Geometry: final body of the model. Coordinates: model frame, mm. Face numbers are marked on the shaded views. A direction names the side the tool comes from. Round coordinates to 2 decimals unless told otherwise and drop trailing zeros. Write each loop counter-clockwise with the first axis right and the second up, starting at its lowest first coordinate (ties: lowest second). Pieces come first, ordered by that corner, then holes. Notation, with made-up numbers: (41, 7) -> (49, 7) arc R28 ccw to (49, 37) -> close; hole circle Ø8 at (81, 39.25). An arc over 180 degrees is marked (long way). One line per item, written item: value. Start each with the question number.
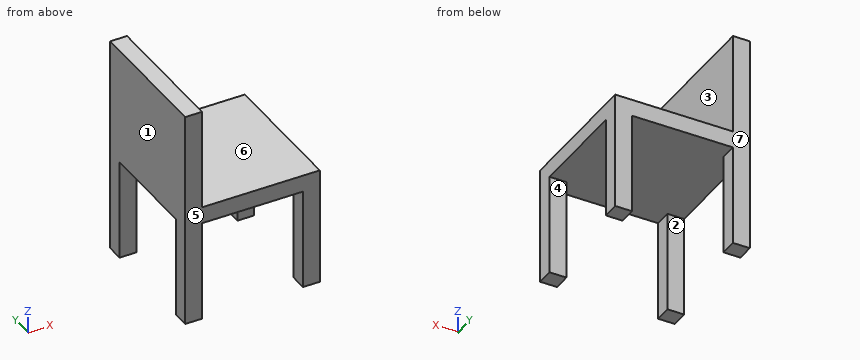
from build123d import *

# Parameters (mm, degrees)
F0_W     = 101.6
F0_H     = 101.6
F1_DEPTH = 12.7
F2_W     = 12.7
F2_H     = 12.7
F3_DEPTH = 76.2
F4_W     = 12.7
F4_H     = 101.6
F5_DEPTH = 76.2


with BuildPart() as f1:
    # F0 (on Top) → F1 (new body)
    with BuildSketch(Plane.XY):
        with Locations((-50.8, 51.606577)):
            Rectangle(F0_W, F0_H)
    extrude(amount=F1_DEPTH)

    # F2 (on face) → F3 (join)
    with BuildSketch(Plane(origin=(0, 0, 0), x_dir=(1, 0, 0), z_dir=(0, 0, -1))):
        with Locations((-95.25, -7.156577)):
            Rectangle(F2_W, F2_H)
        with Locations((-6.35, -7.156577)):
            Rectangle(F2_W, F2_H)
        with Locations((-6.35, -96.056577)):
            Rectangle(F2_W, F2_H)
        with Locations((-95.25, -96.056577)):
            Rectangle(F2_W, F2_H)
    extrude(amount=F3_DEPTH)

    # F4 (on face) → F5 (join)
    with BuildSketch(Plane.XY.offset(12.7)):
        with Locations((-95.25, 51.606577)):
            Rectangle(F4_W, F4_H)
    extrude(amount=F5_DEPTH)


solid = f1.part
(1) Section query D-D (z = 14.5). Output: boundary loops of the cut face in (x, y), and give its area (3 significant figures).
(2) Pull-direction query (Y, two-part tool) for the marked faces 4, 5, 6 and 7; classes: pulls with the +Y half, pulls with the -Y half, needs draft (parallel to the pull), parting line crosses it, or undercut.
(3) Section query C-C (y = 20). Output: boundary loops of the cut face in (x, z).
(4) Section query A-A (z = -33). Output: boundary loops of the cut face in (x, y), and give its area (3 significant figures).
(5) Section query B-B (x = -7). Output: boundary loops of the cut face in (y, z).
(6) Pin query (flat end, axial travel): pin 1 (5 mm diameter, centred on y = 29.5, z = 25, fed in from +X); pin 2 (1.5 mm diameter, centred on x = -79.5, y = 51, fed in from +Z). Return the tip coordinate at first contact, or that it passes through.
(7) Line query: probe 1 along Y at (x, z) = (-95.5, -10.5); probe 2 along X at (y, z) = (97, -60); probe 3 along Z at (x, y) = (-91, 78.5). Output: solid intervals per line, ascending.
(8) Set-up query: the marked faces 1, 2 and 3. Return all of +Z, -Z, +X, -X, +Y, -Y with unobstructed straight access to the full face (end or side cutting, diameter ignored); none if empty.
Results list:
1. outline: (-101.6, 0.81) -> (-88.9, 0.81) -> (-88.9, 102.41) -> (-101.6, 102.41) -> close
1. area: 1,290 mm^2
2. face 4: undercut
2. face 5: pulls with the -Y half
2. face 6: needs draft
2. face 7: pulls with the +Y half
3. outline: (-101.6, 0) -> (0, 0) -> (0, 12.7) -> (-88.9, 12.7) -> (-88.9, 88.9) -> (-101.6, 88.9) -> close
4. outline: (-101.6, 0.81) -> (-88.9, 0.81) -> (-88.9, 13.51) -> (-101.6, 13.51) -> close; (-101.6, 89.71) -> (-88.9, 89.71) -> (-88.9, 102.41) -> (-101.6, 102.41) -> close; (-12.7, 0.81) -> (0, 0.81) -> (0, 13.51) -> (-12.7, 13.51) -> close; (-12.7, 89.71) -> (0, 89.71) -> (0, 102.41) -> (-12.7, 102.41) -> close
4. area: 645 mm^2
5. outline: (0.81, -76.2) -> (13.51, -76.2) -> (13.51, 0) -> (89.71, 0) -> (89.71, -76.2) -> (102.41, -76.2) -> (102.41, 12.7) -> (0.81, 12.7) -> close
6. pin 1: stops at x = -88.9
6. pin 2: stops at z = 12.7
7. probe 1: y = 0.81 to 13.51, 89.71 to 102.41
7. probe 2: x = -101.6 to -88.9, -12.7 to 0
7. probe 3: z = 0 to 88.9
8. face 1: +Z, -Z, -X, +Y, -Y
8. face 2: -Z, +X, -X
8. face 3: +Z, +X, +Y, -Y
